```python
from build123d import *

# Parameters (mm, degrees)
F0_W     = 145
F0_H     = 12.7
F1_DEPTH = 6.35
F3_D     = 5.334
F3_DEPTH = 12.7


with BuildPart() as f1:
    # F0 (on Front) → F1 (new body)
    with BuildSketch(Plane.XZ):
        with Locations((72.5, 6.35)):
            Rectangle(F0_W, F0_H)
    extrude(amount=F1_DEPTH)

    # F3
    with Locations(Plane.XY.offset(12.7)):
        with Locations((12.7, -3.175), (132.3, -3.175)):
            Hole(F3_D / 2, depth=F3_DEPTH)


solid = f1.part
```
The listing builds one solid part. Answer for the finished solid, in the listing's coordinates (mm). Give positions to 0.01 mm unless a question says otherwise; leave off trailing zeros. Order: outer loops, then holes, each group sorted by start corner. A loop starts at its lowest first (then second) coordinate and runs counter-clockwise, first axis right, second up.
Item 1: The part is cut by section A-A, the plane x = 132.3. Give the vertices of the cut face in (y, z), and give its area (3 significant figures).
From the geometry:
outline: (-6.35, 0) - (-5.84, 0) - (-5.84, 12.7) - (-6.35, 12.7) - close; (-0.51, 0) - (0, 0) - (0, 12.7) - (-0.51, 12.7) - close
area: 12.9 mm2
Item 2: The part is cut by section B-B, the plane z = 9.75. Give the vertices of the cut face in (x, y) (3 decimals).
From the geometry:
outline: (0, -6.35) - (145, -6.35) - (145, 0) - (0, 0) - close; hole circle Ø5.334 at (12.7, -3.175); hole circle Ø5.334 at (132.3, -3.175)
Item 3: For a pull along Y with two mould halves and no side action, classify faces 1 (the face through (71, -3, 12.7)), 2 (the face through (134.964, -3.058, 6.261)), 3 (the face through (71, -6.35, 6)) as pulls with the +Y half, pulls with the -Y half, needs draft (parallel to the pull), parting line crosses it, or undercut.
From the geometry:
face 1: needs draft
face 2: undercut
face 3: pulls with the -Y half
Item 4: Find the intervals of material crossed by probe 1 along Y at (x, z) = (12.7, 8.5); probe 2 along X at (y, z) = (-3.5, 2.25); probe 3 along X at (y, z) = (-5, 8.25), in increasing order.
From the geometry:
probe 1: y = -6.35 to -5.84, -0.51 to 0
probe 2: x = 0 to 10.05, 15.35 to 129.65, 134.95 to 145
probe 3: x = 0 to 10.76, 14.64 to 130.36, 134.24 to 145
Item 5: Given pin 1 Ø4 at (x, z) = (125, 10.5) entering from +Y, flat-ended and moving along its own axis, determine where the tip first touches the part or whether it passes through.
From the geometry:
pin 1: stops at y = 0
